Can you work these out from the model? Positions are in its coordinate system, mm. A direction names the side the tool comes from. Round coordinates to 2 decimals unless told otherwise and drop trailing zeros. Order: outer loops, then holes, each group sorted by start corner. A loop starts at its lowest first (then second) coordinate and runs counter-clockwise, first axis right, second up.
Q1. For faces 1 (the face through (1078, -2, 7.4)), 2 (the face through (-15, 7.4, 2)), 3 (the face through (546.41, -2.17, -9.76)), 4 (the face through (1068, 0, 8.2)), which set-ups out of +Z, -Z, +X, -X, +Y, -Y let a thin tool reach every point of the face, with its end or its side?
Q2. If I drill on line 1 (X direction, y = 8.25, z = -5.5); line 2 (X direction, y = -8, z = 2.5); line 3 (Z direction, x = 989, y = 6.5), over which ranges is the centre line in solid material (lowest first)?
Q3. Will these pins go through, and if not, where does the flat tip stop? P1, Ø1, axis at y = -1, z = 9, coming from the +X side; P2, Ø1, axis at x = 808.5, y = -5, coming from the -Z side; P3, Ø1.5, axis at x = 561, y = 5, coming from the +Z side.
Q4. If we section it at A-A (x = 52.5): Please give me the cut outline in (y, z).
Autodesk Inventor part; units mm, degrees
ref_plane "FSS_XY" through (-15, 0, 0) normal (1, 0, 0) x (0, 0, -1)
ref_plane "FSS_YZ" through (-15, 0, 0) normal (0, 0, -1) x (0, 1, 0)
ref_plane "FSS_ZX" through (-15, 0, 0) normal (0, 1, 0) x (1, 0, 0)
sketch "Sketch_1" plane through (0, 0, 0) normal (0, 0, 1) x (1, 0, 0)
  line L0 (1068, 0) -> (10, 0)
  line L1 (10, 0) -> (10, 10)
  line L2 (10, 10) -> (1068, 10)
  line L3 (1068, 10) -> (1068, 0)
  line L4 (1068, 0) -> (10, 0)
revolve "Revolution1" add sketch "Sketch_1" angle 360 about axis through (1068, 0, 0) along (1, 0, 0)
thread "Thread1"
sketch "Sketch_10" plane through (0, 0, 0) normal (0, 1, 0) x (-1, 0, 0)
  line L0 (-10, 0) -> (75, 0)
  line L1 (75, 0) -> (75, -5.3333)
  line L2 (75, -5.3333) -> (74.3333, -6)
  line L3 (74.3333, -6) -> (55, -6)
  line L4 (55, -6) -> (55, -6.8865)
  line L5 (55, -6.8865) -> (54.3865, -7.5)
  line L6 (54.3865, -7.5) -> (15, -7.5)
  line L7 (15, -7.5) -> (15, -9)
  line L8 (15, -9) -> (14, -10)
  line L9 (14, -10) -> (-9.8, -10)
  line L10 (-9.8, -10) -> (-9.8, -8)
  line L11 (-9.8, -8) -> (-10, -8)
  line L12 (-10, -8) -> (-10, 0)
  line L13 (-10, 0) -> (75, 0)
revolve "Revolution2" add sketch "Sketch_10" angle 360 about axis through (10, 0, 0) along (1, 0, 0)
thread "Thread2"
sketch "Sketch_11" plane through (0, 0, 8) normal (0, 0, 1) x (1, 0, 0)
  line L0 (-9, -10) -> (0, -10)
  line L1 (0, -10) -> (0, 10)
  line L2 (0, 10) -> (-9, 10)
  line L3 (-9, 10) -> (-9, -10)
extrude "Extrusion1" cut sketch "Sketch_11" along normal blind 4
sketch "Sketch_12" plane through (0, 0, -8) normal (0, 0, 1) x (1, 0, 0)
  line L0 (-9, -10) -> (0, -10)
  line L1 (0, -10) -> (0, 10)
  line L2 (0, 10) -> (-9, 10)
  line L3 (-9, 10) -> (-9, -10)
extrude "Extrusion2" cut sketch "Sketch_12" against normal blind 4
sketch "Sketch_16" plane through (0, 0, 0) normal (0, 0, 1) x (1, 0, 0)
  line L0 (1091, 0) -> (1068, 0)
  line L1 (1068, 0) -> (1068, 8)
  line L2 (1068, 8) -> (1068.2, 8)
  line L3 (1068.2, 8) -> (1068.2, 10)
  line L4 (1068.2, 10) -> (1077, 10)
  line L5 (1077, 10) -> (1078, 9)
  line L6 (1078, 9) -> (1078, 7.5)
  line L7 (1078, 7.5) -> (1087, 7.5)
  line L8 (1087, 7.5) -> (1087, 7.15)
  line L9 (1087, 7.15) -> (1088.15, 7.15)
  line L10 (1088.15, 7.15) -> (1088.15, 7.5)
  line L11 (1088.15, 7.5) -> (1090.25, 7.5)
  line L12 (1090.25, 7.5) -> (1091, 6.75)
  line L13 (1091, 6.75) -> (1091, 0)
  line L14 (1091, 0) -> (1068, 0)
revolve "Revolution3" add sketch "Sketch_16" angle 360 about axis through (1091, 0, 0) along (1, 0, 0)
ref_plane "FSS_XY" through (-15, 0, 0) normal (1, 0, 0) x (0, 0, -1)
ref_plane "FSS_YZ" through (-15, 0, 0) normal (0, 0, -1) x (0, 1, 0)
ref_plane "FSS_ZX" through (-15, 0, 0) normal (0, 1, 0) x (1, 0, 0)
ref_plane "SSS_XY" through (1078, 0, 0) normal (1, 0, 0) x (0, 0, -1)
ref_plane "SSS_YZ" through (1078, 0, 0) normal (0, 0, -1) x (0, 1, 0)
ref_plane "SSS_ZX" through (1078, 0, 0) normal (0, 1, 0) x (1, 0, 0)
ref_plane "bnt_s_1_XY" through (0, 0, 0) normal (-1, 0, 0) x (0, 0, -1)
ref_plane "bnt_s_1_YZ" through (0, 0, 0) normal (0, 0, -1) x (0, -1, 0)
ref_plane "bnt_s_1_ZX" through (0, 0, 0) normal (0, -1, 0) x (-1, 0, 0)
properties part number "BNT 2010-2.61000-J1K Shaft"
Solution:
1. face 1: +X
1. face 2: -X
1. face 3: +X, -X
1. face 4: none
2. line 1: x = -14.08 to 9.8, 10 to 1068, 1068.2 to 1077.08
2. line 2: x = -15 to 9.8, 10 to 1068, 1068.2 to 1078
2. line 3: z = -7.6 to 7.6
3. P1: stops at x = 1078
3. P2: stops at z = -8.93
3. P3: stops at z = 9.05
4. outline: circle Ø20 at (0, 0)
